from build123d import *

# Parameters (mm, degrees)
F0_W     = 170
F0_H     = 360
F1_DEPTH = 30
F2_R     = 10
F3_DEPTH = 30.001
F4_R     = 76
F4_R_2   = 10
F5_DEPTH = 25


with BuildPart() as f1:
    # F0 (on Top) → F1 (new body)
    with BuildSketch(Plane.XY):
        Rectangle(F0_W, F0_H)
    extrude(amount=F1_DEPTH)

    # F2 (on face) → F3 (cut, through all)
    with BuildSketch(Plane.XY.offset(30)):
        with Locations((0, -95)):
            Circle(F2_R)
    extrude(amount=-F3_DEPTH, mode=Mode.SUBTRACT)

    # F4 (on face) → F5 (cut)
    with BuildSketch(Plane.XY.offset(30)):
        with Locations((0, -95)):
            Circle(F4_R)
        with Locations((0, -95)):
            Circle(F4_R)
        with Locations((0, -95)):
            Circle(F4_R_2, mode=Mode.SUBTRACT)
    extrude(amount=-F5_DEPTH, mode=Mode.SUBTRACT)


solid = f1.part
Geometry: final body of the model. Coordinates: model frame, mm. A direction names the side the tool comes from. Round coordinates to 2 decimals unless told otherwise and drop trailing zeros. Order: outer loops, then holes, each group sorted by start corner. A loop starts at its lowest first (then second) coordinate and runs counter-clockwise, first axis right, second up.
Q1. Mould query, pull axis Y, two halves, no side actions, for faces 1 (the face through (40.86, -30.92, 17.68)), 2 (the face through (-1, 180, 15)), 3 (the face through (-1, -180, 15)). Classes: released by +Y, released by -Y, zero draft, split by the parting line, or undercut.
Result sheet:
face 1: undercut
face 2: released by +Y
face 3: released by -Y
Q2. Section B-B, the plane y = -95. Output: boundary loops of the cut face in (x, z), and give its area (3 significant figures).
Result sheet:
outline: (-85, 0) - (-10, 0) - (-10, 5) - (-76, 5) - (-76, 30) - (-85, 30) - close; (10, 0) - (85, 0) - (85, 30) - (76, 30) - (76, 5) - (10, 5) - close
area: 1,200 mm2
Q3. Material intervals for probe 1 along Y at (x, z) = (0, 1.9); probe 2 along Y at (x, z) = (0, 10.5); probe 3 along Z at (x, y) = (44, -148), sorted ascending.
Result sheet:
probe 1: y = -180 to -105, -85 to 180
probe 2: y = -180 to -171, -19 to 180
probe 3: z = 0 to 5
Q4. Section D-D, the plane x = 30.5. Output: boundary loops of the cut face in (y, z).
Result sheet:
outline: (-180, 0) - (180, 0) - (180, 30) - (-25.39, 30) - (-25.39, 5) - (-164.61, 5) - (-164.61, 30) - (-180, 30) - close
Q5. Access query for faces 4 (the face through (-85, -3, 15)), 5 (the face through (-1, -111, 5)). Directions: +Z, -Z, +X, -X, +Y, -Y. A direction counts if a zero-diameter tool reaches every point of the face in a straight line with its end or side. Return the directions, or none.
Result sheet:
face 4: +Z, -Z, -X, +Y, -Y
face 5: +Z
Q6. Section A-A, the plane x = 0. Output: boundary loops of the cut face in (y, z), and give its area (3 significant figures).
Result sheet:
outline: (-180, 0) - (-105, 0) - (-105, 5) - (-171, 5) - (-171, 30) - (-180, 30) - close; (-85, 0) - (180, 0) - (180, 30) - (-19, 30) - (-19, 5) - (-85, 5) - close
area: 6,900 mm2
Q7. Section C-C, the plane z = 17.25. Output: boundary loops of the cut face in (x, y), and give its area (3 significant figures).
Result sheet:
outline: (-85, -180) - (85, -180) - (85, 180) - (-85, 180) - close; hole circle Ø152 at (0, -95)
area: 43,100 mm2
